from build123d import *

# Parameters (mm, degrees)
CROQUIS1_W              = 51
CROQUIS1_H              = 51
SALIENTE_EXTRUIR1_DEPTH = 1.6
REDONDEO1_R             = 5
CROQUIS2_W              = 4
CROQUIS2_H              = 4
CROQUIS2_W_2            = 8
CROQUIS2_H_2            = 8
SALIENTE_EXTRUIR2_DEPTH = 1
CROQUIS3_R              = 1.25
CORTAR_EXTRUIR1_DEPTH   = 37.097922378
CROQUIS4_W              = 4.75
CROQUIS4_H              = 4.75
SALIENTE_EXTRUIR3_DEPTH = 0.25
CROQUIS5_R              = 0.75
CORTAR_EXTRUIR2_DEPTH   = 37.109867073
CROQUIS6_R              = 3.5
SALIENTE_EXTRUIR4_DEPTH = 12
REDONDEO2_R             = 0.5
CROQUIS7_W              = 38.1
CROQUIS7_H              = 2.54
SALIENTE_EXTRUIR5_DEPTH = 8
CROQUIS8_R              = 0.512123022
SALIENTE_EXTRUIR6_DEPTH = 0.25


with BuildPart() as part:
    # Croquis1 → Saliente-Extruir1 (new body)
    with BuildSketch(Plane(origin=(0, 0, 0), x_dir=(1, 0, 0), z_dir=(0, 1, 0))):
        Rectangle(CROQUIS1_W, CROQUIS1_H)
    extrude(amount=-SALIENTE_EXTRUIR1_DEPTH)

    # Redondeo1
    redondeo1_edges = [part.edges().sort_by_distance(p)[0] for p in [
        (25.5, -0.8, 25.5),
        (-25.5, -0.8, 25.5),
        (-25.5, -0.8, -25.5),
        (25.5, -0.8, -25.5),
    ]]
    fillet(redondeo1_edges, radius=REDONDEO1_R)

    # Croquis2 → Saliente-Extruir2 (add)
    with BuildSketch(Plane(origin=(0, 0, 0), x_dir=(1, 0, 0), z_dir=(0, 1, 0))):
        with Locations((-10.387074195, 0.047356258)):
            Rectangle(CROQUIS2_W, CROQUIS2_H)
        with Locations((7.8, 5.359014033)):
            Rectangle(CROQUIS2_W_2, CROQUIS2_H_2)
    extrude(amount=SALIENTE_EXTRUIR2_DEPTH)

    # Croquis3 → Cortar-Extruir1 (cut, through all)
    with BuildSketch(Plane(origin=(0, 0, 0), x_dir=(1, 0, 0), z_dir=(0, 1, 0))):
        with Locations(Location((-22.25, 22.25, 0), (0, 0, 270))):
            Circle(CROQUIS3_R)
        with Locations(Location((-22.25, -22.25, 0), (0, 0, 270))):
            Circle(CROQUIS3_R)
        with Locations(Location((22.25, -22.25, 0), (0, 0, 270))):
            Circle(CROQUIS3_R)
        with Locations(Location((22.25, 22.25, 0), (0, 0, 270))):
            Circle(CROQUIS3_R)
    extrude(amount=-CORTAR_EXTRUIR1_DEPTH, mode=Mode.SUBTRACT)

    # Croquis4 → Saliente-Extruir3 (add)
    with BuildSketch(Plane(origin=(0, 0, 0), x_dir=(1, 0, 0), z_dir=(0, 1, 0))):
        with Locations((-3.48, -22.2)):
            Rectangle(CROQUIS4_W, CROQUIS4_H)
        with Locations((6.42, -22.2)):
            Rectangle(CROQUIS4_W, CROQUIS4_H)
        with Locations((15.72, -22.2)):
            Rectangle(CROQUIS4_W, CROQUIS4_H)
        with Locations((-10.52, -21.7)):
            Rectangle(CROQUIS4_W, CROQUIS4_H)
        with Locations((-17.12, -21.7)):
            Rectangle(CROQUIS4_W, CROQUIS4_H)
    extrude(amount=SALIENTE_EXTRUIR3_DEPTH)

    # Croquis5 → Cortar-Extruir2 (cut, through all)
    with BuildSketch(Plane(origin=(0, 0.25, 0), x_dir=(1, 0, 0), z_dir=(0, 1, 0))):
        with Locations(Location((-3.48, -22.2, 0), (0, 0, 270))):
            Circle(CROQUIS5_R)
        with Locations(Location((6.42, -22.2, 0), (0, 0, 270))):
            Circle(CROQUIS5_R)
        with Locations(Location((15.72, -22.2, 0), (0, 0, 270))):
            Circle(CROQUIS5_R)
    extrude(amount=-CORTAR_EXTRUIR2_DEPTH, mode=Mode.SUBTRACT)

    # Croquis6 → Saliente-Extruir4 (add)
    with BuildSketch(Plane(origin=(0, -1.6, 0), x_dir=(1, 0, 0), z_dir=(0, 1, 0))):
        with Locations(Location((-16.236720917, 22.626792328, 0), (0, 0, 270))):
            Circle(CROQUIS6_R)
        with Locations(Location((16.410663599, 22.626792328, 0), (0, 0, 270))):
            Circle(CROQUIS6_R)
    extrude(amount=-SALIENTE_EXTRUIR4_DEPTH)

    # Redondeo2
    redondeo2_edges = [part.edges().sort_by_distance(p)[0] for p in [
        (-16.236720917, -13.6, -26.126792328),
        (16.410663599, -13.6, -26.126792328),
    ]]
    fillet(redondeo2_edges, radius=REDONDEO2_R)

    # Croquis7 → Saliente-Extruir5 (add)
    with BuildSketch(Plane.XZ.offset(1.6)):
        with Locations((-3.45, -17.29)):
            Rectangle(CROQUIS7_W, CROQUIS7_H)
        with Locations((-3.45, 8.06)):
            Rectangle(CROQUIS7_W, CROQUIS7_H)
    extrude(amount=SALIENTE_EXTRUIR5_DEPTH)

    # Croquis8 → Saliente-Extruir6 (add)
    with BuildSketch(Plane(origin=(0, 1, 0), x_dir=(1, 0, 0), z_dir=(0, 1, 0))):
        with Locations(Location((-10.387074195, 0, 0), (0, 0, 270))):
            Circle(CROQUIS8_R)
    extrude(amount=SALIENTE_EXTRUIR6_DEPTH)


solid = part.part
Model file for the job. Use its own axes, mm. A direction names the side the tool comes from. Give positions to 0.01 mm unless a question says otherwise; leave off trailing zeros. Write each loop counter-clockwise with the first axis right and the second up, starting at its lowest first coordinate (ties: lowest second). Pieces come first, ordered by that corner, then holes. Notation, with made-up numbers: (16, 76.25) -> (57, 76.25) arc R22 cw to (57, 99.25) -> close; hole circle Ø7 at (26, 12). An arc over 180 degrees is marked (long way). Write item = value, one per line.
(1) Slice it at A-A, the plane x = -3.48. Give the cut face in (y, z) (3 decimals).
Determined:
outline = (-9.6, -18.56) -> (-1.6, -18.56) -> (-1.6, -25.5) -> (0, -25.5) -> (0, 19.825) -> (0.25, 19.825) -> (0.25, 21.45) -> (-1.6, 21.45) -> (-1.6, 9.33) -> (-9.6, 9.33) -> (-9.6, 6.79) -> (-1.6, 6.79) -> (-1.6, -16.02) -> (-9.6, -16.02) -> close; (-1.6, 22.95) -> (0.25, 22.95) -> (0.25, 24.575) -> (0, 24.575) -> (0, 25.5) -> (-1.6, 25.5) -> close
(2) Slice it at C-C, the plane y = -4.75. Give the cut face in (x, z), then the cut area to 3 significant figures.
Determined:
outline = (-22.5, -18.56) -> (15.6, -18.56) -> (15.6, -16.02) -> (-22.5, -16.02) -> close; (-22.5, 6.79) -> (15.6, 6.79) -> (15.6, 9.33) -> (-22.5, 9.33) -> close; circle Ø7 at (-16.24, -22.63); circle Ø7 at (16.41, -22.63)
area = 271 mm2
(3) Tool access for faces 1 (the face through (-4, -6, -16.02)), 2 (the face through (-11, 0.25, 22)), 3 (the face through (-17.577, -7.27, -19.394)), 4 (the face through (-4, -6, 9.33)): list every direction of +Z, -Z, +X, -X, +Y, -Y with a clear straight run to the whole face (end or side of a thin tool).
Determined:
face_1 = +X, -X, -Y
face_2 = +Z, +X, -X, +Y
face_3 = -Y
face_4 = +Z, +X, -X, -Y
(4) Probe line 1 along Z through (x, y) = (-6, -5.5); line 2 along X through (y, z) = (-1.15, 22.25); line 3 along X through (y, z) = (-1.2, -22.25). List the from-to ranges inside material, lowest first.
Determined:
line_1 = -18.56 to -16.02, 6.79 to 9.33
line_2 = -25.18 to -23.5, -21 to -4.23, -2.73 to 5.67, 7.17 to 14.97, 16.47 to 21, 23.5 to 25.18
line_3 = -25.18 to -23.5, -21 to 21, 23.5 to 25.18
(5) Slice it at B-B, the plane x = 6.42. Give the cut face in (y, z) (3 decimals), then the cut area to 3 significant figures.
Determined:
outline = (-9.6, -18.56) -> (-1.6, -18.56) -> (-1.6, -25.5) -> (0, -25.5) -> (0, -9.359) -> (1, -9.359) -> (1, -1.359) -> (0, -1.359) -> (0, 19.825) -> (0.25, 19.825) -> (0.25, 21.45) -> (-1.6, 21.45) -> (-1.6, 9.33) -> (-9.6, 9.33) -> (-9.6, 6.79) -> (-1.6, 6.79) -> (-1.6, -16.02) -> (-9.6, -16.02) -> close; (-1.6, 22.95) -> (0.25, 22.95) -> (0.25, 24.575) -> (0, 24.575) -> (0, 25.5) -> (-1.6, 25.5) -> close
area = 129 mm2
(6) Slice it at D-D, the plane z = 22.2. Give the number of separate pieces and of enclosed holes in the cut face, then the cut area to 3 significant figures.
Determined:
separate_pieces = 6
enclosed_holes = 0
area = 70.3 mm2
(7) Flat gauge pins, fed straight in: P1, Ø2, axis at x = -13, y = -6.5, coming from the +Z side; P2, Ø3, axis at x = 6.5, y = -9.5, coming from the -Z side; P3, Ø2, axis at y = -3.5, z = 8.5, coming from the -X side. Where does each tip first touch, or does it go through?
Determined:
P1 = 9.33
P2 = -18.56
P3 = -22.5
